Build history of the part. All positions in model axes, mm. Face numbers are marked on the shaded views. A direction names the side the tool comes from. Give positions to 0.01 mm unless a question says otherwise; leave off trailing zeros. Loops run counter-clockwise (first coordinate to the right, second up) from the corner with the lowest first, then second, coordinate; pieces in that order, holes last. Notation, with made-up numbers: (57, -10) -> (90, -10) arc R11 ccw to (90, -6) -> close; hole circle Ø4 at (39, -4). An arc over 180 degrees is marked (long way). Answer as a JSON object with one key per item and string values. Group by question number.
Autodesk Inventor part; units mm, degrees
ref_plane "YZ Plane" through (0, 0, 0) normal (1, 0, 0) x (0, 1, 0)
ref_plane "XZ Plane" through (0, 0, 0) normal (0, 1, 0) x (-1, 0, 0)
ref_plane "XY Plane" through (0, 0, 0) normal (0, 0, 1) x (1, 0, 0)
sketch "Szkic1" plane through (0, 0, 0) normal (0, 1, 0) x (-1, 0, 0)
  line L0 (0, 0) -> (0, -100)
  line L1 (0, -100) -> (-65, -100)
  line L2 (-65, -100) -> (-65, 0)
  line L3 (-65, 0) -> (0, 0)
  dimension "d0" = 100
  dimension "d1" = 65
extrude "Wyciągnięcie proste1" add sketch "Szkic1" along normal blind 15
sketch "Szkic3" plane through (0, 0, 0) normal (0, -1, 0) x (1, 0, 0)
  line L0 (0, 0) -> (65, 0)
  line L1 (32.5, 0) -> (32.5, -100)
  line L2 (65, -100) -> (0, -100)
  line L3 (32.5, -50) -> (15, -50)
  line L4 (15, -50) -> (50, -50)
  line L5 (50, -50) -> (50, 0)
  line L6 (65, 0) -> (65, -100)
  line L7 (50, 0) -> (65, 0)
  line L8 (65, 0) -> (65, -100)
  line L9 (65, -100) -> (50, -100)
  line L10 (50, -100) -> (50, -50)
  line L11 (15, -50) -> (15, -100)
  line L12 (15, -100) -> (0, -100)
  line L13 (0, -100) -> (0, 0)
  line L14 (0, -100) -> (0, 0)
  line L15 (0, 0) -> (15, 0)
  line L16 (15, -50) -> (15, 0)
  dimension "d4" = 17.5
  dimension "d5" = 35
extrude "Wyciągnięcie proste2" add sketch "Szkic3" along normal blind 10 contours L0 L16 L11 L2 L13 | L0 L6 L2 L10 L5
fillet "Zaokrąglenie1" radius 6 4 edges at (15, -5, -100) (15, -5, 0) (50, -5, 0) (50, -5, -100)
sketch "Szkic4" plane through (0, 15, 0) normal (0, 1, 0) x (1, 0, 0)
  line L0 (0, 0) -> (0, 35)
  line L1 (0, 0) -> (0, 100)
  line L2 (0, 35) -> (65, 35)
  line L3 (65, 100) -> (65, 0)
  line L4 (0, 0) -> (65, 0)
  line L5 (65, 0) -> (65, 35)
  line L6 (0, 0) -> (65, 0)
  line L7 (9, 0) -> (56, 0)
  dimension "d9" = 35
extrude "Wyciągnięcie proste3" add sketch "Szkic4" along normal blind 10
sketch "Szkic5" plane through (0, 25, 0) normal (0, 1, 0) x (1, 0, 0)
  line L0 (0, 0) -> (32.5, 0)
  line L1 (9, 0) -> (56, 0)
  line L2 (32.5, 0) -> (32.5, 100)
  line L3 (56, 100) -> (9, 100)
  line L4 (0, 35) -> (65, 35)
  line L5 (32.5, 35) -> (10, 35)
  line L6 (10, 35) -> (55, 35)
  line L7 (55, 35) -> (55, 0)
  line L8 (10, 35) -> (10, 0)
  line L9 (10, 35) -> (16.1714, 0)
  line L10 (10, 35) -> (45.5399, 35) construction
  line L11 (55, 35) -> (48.8286, 0)
  line L12 (55, 35) -> (90.5399, 35) construction
  line L13 (65, 0) -> (65, 35)
  line L14 (55, 0) -> (65, 0)
  line L15 (65, 0) -> (65, 35)
  line L16 (55, 35) -> (65, 35)
  line L17 (10, 35) -> (0, 35)
  line L18 (0, 35) -> (0, 0)
  line L19 (0, 0) -> (10, 0)
  line L20 (9, 0) -> (0, 0)
  line L21 (0, 0) -> (0, 35)
  line L22 (0, 0) -> (0, 100)
  dimension "d12" = 22.5
  dimension "d13" = 45
  dimension "d14" = 80
  dimension "d15" = 100
extrude "Wyciągnięcie proste4" add sketch "Szkic5" along normal blind 8 contours L18 L4 L8 L0 | L8 L9 L0 | L4 L13 L14 L1 L7 | L7 L1 L11
sketch "Szkic6" plane through (0, 15, 0) normal (0, 1, 0) x (1, 0, 0)
  line L0 (56, 100) -> (9, 100)
  line L1 (32.5, 100) -> (32.5, 0)
  line L2 (32.5, 0) -> (32.5, 50)
  line L3 (32.5, 50) -> (0, 50)
  line L4 (0, 0) -> (0, 100)
  line L5 (32.5, 50) -> (65, 50)
  line L6 (65, 35) -> (65, 100)
  circle A0 centre (32.5, 50) radius 27.0416
  point P0 (10, 35)
extrude "Wyciągnięcie proste5" cut sketch "Szkic6" along normal blind 15 and the other way blind 4
chamfer "Faza1" distance 6 angle 45 1 edges at (32.5, 25, -22.9584)
sketch "Szkic7" plane through (0, 0, 0) normal (0, -1, 0) x (1, 0, 0)
  line L0 (16.1714, 0) -> (48.8286, 0)
  line L1 (32.5, 0) -> (32.5, -100)
  line L2 (65, -100) -> (0, -100)
  line L3 (32.5, -50) -> (0, -50)
  line L4 (0, -50) -> (0, -87)
  line L5 (0, -100) -> (0, -35)
  line L6 (0, -87) -> (32.5, -87)
  circle A0 centre (32.5, -50) radius 8
  circle A1 centre (32.5, -87) radius 8
  line L7 (40.5, -50) -> (40.5, -87)
  line L8 (24.5, -87) -> (24.5, -50)
  point P0 (0, 0)
  dimension "d25" = 37
  dimension "d26" = 16
  dimension "d27" = 16
extrude "Wyciągnięcie proste6" cut sketch "Szkic7" against normal blind 15 contours A0 L1 | L1 L3 A0 | L1 A0 L3 | L7 A1 L1 A0 | A0 L1 A1 L8 | A1 L1 | A1 L1 L6 | L6 L1 A1
fillet "Zaokrąglenie2" radius 6 2 edges at (24.5, 13, -75.8312) (40.5, 13, -75.8312)
sketch "Szkic8" plane through (0, 33, 0) normal (0, 1, 0) x (1, 0, 0)
  line L0 (55, 35) -> (48.8286, 0)
  line L1 (51.9929, 17.9457) -> (57.9017, 16.9038)
  line L2 (51.9929, 17.9457) -> (57.9929, 17.9457) construction
  line L3 (57.9017, 16.9038) -> (61.0926, 35)
  line L4 (65, 35) -> (55, 35)
  line L5 (57.9017, 16.9038) -> (54.9211, 0)
  line L6 (65, 0) -> (56, 0)
  line L7 (48.8286, 0) -> (65, 0)
  line L8 (50.9367, 0) -> (50.9367, 8)
  line L9 (50.9367, 0) -> (58.9367, 0) construction
  line L10 (50.9367, 8) -> (65, 8)
  line L11 (65, 0) -> (65, 35)
  circle A0 centre (56.3317, 8) radius 2.5
  line L12 (56.3317, 8) -> (59.2838, 24.7417)
  circle A1 centre (59.2838, 24.7417) radius 2.5
  line L13 (53.8317, 8) -> (56.8208, 25.1705)
  line L14 (58.8317, 8) -> (61.7448, 24.302)
  point P0 (0, 0)
  dimension "d31" = 6
  dimension "d32" = 10
  dimension "d33" = 8
  dimension "d34" = 90
  dimension "d35" = 5
  dimension "d36" = 17
  dimension "d37" = 5
extrude "Wyciągnięcie proste7" cut sketch "Szkic8" against normal blind 2 contours L13 A1 L3 L1 | L1 L5 A0 L13 | A1 L3 | L3 A1 | L3 A1 L14 A0 L5 | A0 L5 L10 L13 | A0 L10 L5 | L10 L5 A0 | A0 L5 L10
sketch "Szkic9" plane through (0, 33, 0) normal (0, 1, 0) x (1, 0, 0)
  line L0 (16.1714, 0) -> (10, 35)
  line L1 (12.5503, 20.5363) -> (6.6415, 19.4944)
  line L2 (12.5503, 20.5363) -> (18.5503, 20.5363) construction
  line L3 (6.6415, 19.4944) -> (3.9074, 35)
  line L4 (0, 35) -> (10, 35)
  line L5 (6.6415, 19.4944) -> (10.0622, 0.0948)
  line L6 (10.0622, 0.0948) -> (10.0622, 8.0948)
  line L7 (0, 35) -> (0, 0)
  line L8 (8.6516, 8.0948) -> (5.6995, 24.8365)
  circle A0 centre (8.6516, 8.0948) radius 2.5
  circle A1 centre (5.6995, 24.8365) radius 2.5
  line L9 (8.1616, 25.2706) -> (11.1136, 8.5289)
  line L10 (6.1895, 7.6606) -> (3.2375, 24.4024)
  dimension "d40" = 6
  dimension "d41" = 170
  dimension "d42" = 8
  dimension "d43" = 17
  dimension "d44" = 5
  dimension "d45" = 5
extrude "Wyciągnięcie proste8" cut sketch "Szkic9" against normal blind 2 contours L9 A0 L5 L1 | L1 L3 A1 L9 | L5 A0 L10 A1 L3 | A1 L3 | A0 L5 | L3 A1 | L5 A0
sketch "Szkic10" plane through (0, 31, 0) normal (0, 1, 0) x (1, 0, 0)
  arc A0 (8.1616, 25.2706) -> (3.2375, 24.4024) centre (5.6995, 24.8365) ccw
  arc A1 (6.1895, 7.6606) -> (11.1136, 8.5289) centre (8.6516, 8.0948) ccw
  line L0 (5.6995, 24.8365) -> (8.6516, 8.0948)
  circle A2 centre (8.6516, 8.0948) radius 1.5
  circle A3 centre (5.6995, 24.8365) radius 1.5
  arc A4 (53.8317, 8) -> (58.8317, 8) centre (56.3317, 8) ccw
  arc A5 (61.7448, 24.302) -> (56.8208, 25.1705) centre (59.2838, 24.7417) ccw
  line L1 (56.3317, 8) -> (59.2838, 24.7417)
  circle A6 centre (56.3317, 8) radius 1.5
  circle A7 centre (59.2838, 24.7417) radius 1.5
  point P0 (0, 0)
  dimension "d48" = 3
  dimension "d49" = 3
  dimension "d50" = 3
  dimension "d51" = 3
extrude "Wyciągnięcie proste9" cut sketch "Szkic10" against normal blind 41
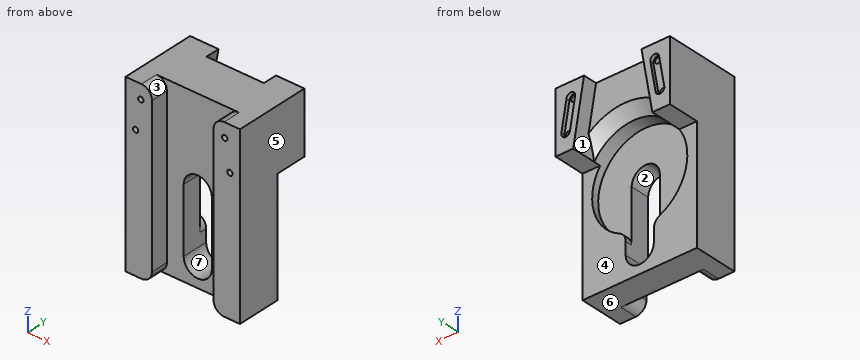
(1) Pin check, flat tips, straight feed: pin 1 (8.5 mm diameter, centred on x = 8.5, z = -12, fed in from +Y); pin 2 (5 mm diameter, centred on x = 60, y = 25.5, fed in from -Z); pin 3 (19.5 mm diameter, centred on x = 23.5, z = -68, fed in from +Y); pin 4 (14 mm diameter, centred on x = 40, z = -61.5, fed in from -Y). Stop position of each tip, or through.
(2) Pull direction Z, two halves, no side cores. Call the marked faces 5, 6 and 7: pulls with the +Z half, pulls with the -Z half, needs draft (parallel to the pull), parting line crosses it, or undercut.
(3) Probe line 1 along X through (y, z) = (-4, -30); line 2 along X through (y, z) = (7.5, -80); line 3 along Z through (x, y) = (28.5, 17.5). List the from-to ranges inside material, lowest first. Write a range as [from, to].
(4) Saw through at B-B on y = -1.5. List the corners of the cut face in (x, z).
(5) Saw through at A-A on x = 32.5. List the corners of the cut face in (y, z), plus the area to 3 significant figures.
(6) 3-axis set-ups, long thin cutter, end or side, ignore diameter. For the marked faces 1, 2, 3 and 4: which of +Z, -Z, +X, -X, +Y, -Y reach the whole face in a straight line?
(7) Saw through at D-D on y = 13.5. List the corners of the cut face in (x, z), plus the area to 3 significant figures.
(8) Saw through at C-C on z = -62.5. List the corners of the cut face in (x, y).
Calculated:
{
 "1": {"pin 1": "stops at y = 33", "pin 2": "stops at z = -35", "pin 3": "stops at y = 15", "pin 4": "stops at y = 0"},
 "2": {"face 5": "needs draft", "face 6": "pulls with the -Z half", "face 7": "undercut"},
 "3": {"line 1": "x = [0, 15], [50, 65]", "line 2": "x = [0, 24.5], [40.5, 65]", "line 3": "z = [-23.26, 0]"},
 "4": {"outline": "(0, -100) -> (9, -100) arc R6 ccw to (15, -94) -> (15, -6) arc R6 ccw to (9, 0) -> (0, 0) -> close; (50, -94) arc R6 ccw to (56, -100) -> (65, -100) -> (65, 0) -> (56, 0) arc R6 ccw to (50, -6) -> close; hole circle Ø3 at (5.7, -24.84); hole circle Ø3 at (8.65, -8.09); hole circle Ø3 at (56.33, -8); hole circle Ø3 at (59.28, -24.74)"},
 "5": {"outline": "(0, -100) -> (15, -100) -> (15, -95) -> (0, -95) -> close; (0, -42) -> (11, -42) -> (11, -22.96) -> (19, -22.96) -> (25, -16.96) -> (25, 0) -> (0, 0) -> close", "area": "840 mm^2"},
 "6": {"face 1": "-Z, +Y", "face 2": "+Y, -Y", "face 3": "+Z, -Y", "face 4": "-Z, +X, -X, +Y"},
 "7": {"outline": "(0, -100) -> (65, -100) -> (65, 0) -> (0, 0) -> close; hole circle Ø3 at (5.7, -24.84); hole circle Ø3 at (8.65, -8.09); hole (21.04, -74.49) arc R6 cw to (24.5, -79.93) -> (24.5, -87) arc R8 ccw to (40.5, -87) -> (40.5, -79.93) arc R6 cw to (43.96, -74.49) arc R27.04 ccw (long way) to start; hole circle Ø3 at (56.33, -8); hole circle Ø3 at (59.28, -24.74)", "area": "3,900 mm^2"},
 "8": {"outline": "(0, -10) -> (15, -10) -> (15, 0) -> (24.5, 0) -> (24.5, 11) -> (8.52, 11) -> (8.52, 15) -> (0, 15) -> close; (40.5, 0) -> (50, 0) -> (50, -10) -> (65, -10) -> (65, 15) -> (56.48, 15) -> (56.48, 11) -> (40.5, 11) -> close"}
}
